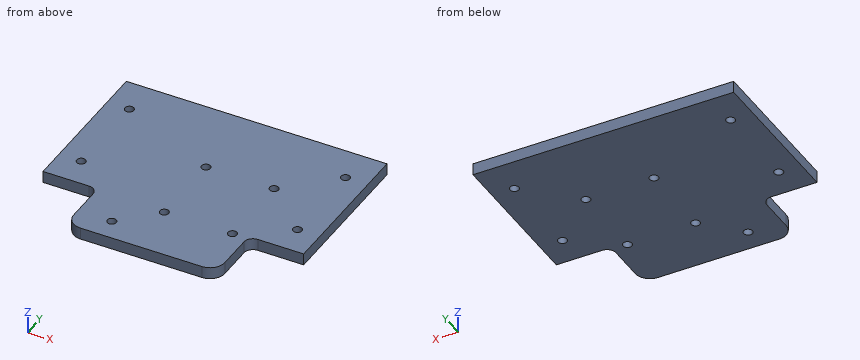
```python
from build123d import *

# Parameters (mm, degrees)
SKETCH_1_W          = 88
SKETCH_1_H          = 72
EXTRUDE_1_DEPTH     = 4
SKETCH_2_W          = 18.5
SKETCH_2_H          = 20
CUT_EXTRUDE_1_DEPTH = 114.771701227
FILLET_1_R          = 3
SKETCH_3_W          = 18.5
SKETCH_3_H          = 20
CUT_EXTRUDE_2_DEPTH = 114.771701227
FILLET_2_R          = 3
SKETCH_5_R          = 1.5
CUT_EXTRUDE_4_DEPTH = 114.771701227
SKETCH_4_R          = 1.5
CUT_EXTRUDE_3_DEPTH = 114.771701227
FILLET_4_R          = 5


with BuildPart() as part:
    # 草图1 → 凸台-拉伸1 (new body)
    with BuildSketch(Plane.XY):
        with Locations((44, 36)):
            Rectangle(SKETCH_1_W, SKETCH_1_H)
    extrude(amount=EXTRUDE_1_DEPTH)

    # 草图2 → 切除-拉伸1 (cut, through all)
    with BuildSketch(Plane.XY.offset(4)):
        with Locations((9.25, 10)):
            Rectangle(SKETCH_2_W, SKETCH_2_H)
    extrude(amount=-CUT_EXTRUDE_1_DEPTH, mode=Mode.SUBTRACT)

    # 圆角1
    fillet_1_edges = [part.edges().sort_by_distance(p)[0] for p in [
        (18.5, 20, 2),
    ]]
    fillet(fillet_1_edges, radius=FILLET_1_R)

    # 草图3 → 切除-拉伸2 (cut, through all)
    with BuildSketch(Plane.XY.offset(4)):
        with Locations((78.75, 10)):
            Rectangle(SKETCH_3_W, SKETCH_3_H)
    extrude(amount=-CUT_EXTRUDE_2_DEPTH, mode=Mode.SUBTRACT)

    # 圆角2
    fillet_2_edges = [part.edges().sort_by_distance(p)[0] for p in [
        (69.5, 20, 2),
    ]]
    fillet(fillet_2_edges, radius=FILLET_2_R)

    # 草图5 → 切除-拉伸4 (cut, through all)
    with BuildSketch(Plane.XY.offset(4)):
        with Locations((80.5, 60)):
            Circle(SKETCH_5_R)
        with Locations((80.5, 30)):
            Circle(SKETCH_5_R)
        with Locations(Location((30, 7.5, 0), (0, 0, 180))):
            Circle(SKETCH_5_R)
        with Locations(Location((7.5, 30, 0), (0, 0, 180))):
            Circle(SKETCH_5_R)
        with Locations(Location((7.5, 60, 0), (0, 0, 180))):
            Circle(SKETCH_5_R)
    extrude(amount=-CUT_EXTRUDE_4_DEPTH, mode=Mode.SUBTRACT)

    # 草图4 → 切除-拉伸3 (cut, through all)
    with BuildSketch(Plane.XY.offset(4)):
        with Locations((41.5, 45)):
            Circle(SKETCH_4_R)
        with Locations((64.5, 45)):
            Circle(SKETCH_4_R)
        with Locations((64.5, 19)):
            Circle(SKETCH_4_R)
        with Locations((41.5, 19)):
            Circle(SKETCH_4_R)
    extrude(amount=-CUT_EXTRUDE_3_DEPTH, mode=Mode.SUBTRACT)

    # 圆角4
    fillet_4_edges = [part.edges().sort_by_distance(p)[0] for p in [
        (18.5, 0, 2),
        (69.5, 0, 2),
    ]]
    fillet(fillet_4_edges, radius=FILLET_4_R)


solid = part.part
```
CAD build for the part. Positions are in the model's coordinates, mm. Round coordinates to 2 decimals unless told otherwise and drop trailing zeros. Order: outer loops, then holes, each group sorted by start corner. A loop starts at its lowest first (then second) coordinate and runs counter-clockwise, first axis right, second up.
Q1. Slice it at D-D (x = 41.5). Write the cut outline in (y, z), and give its area (3 significant figures).
Q2. Slice it at C-C (y = 45). Write the cut outline in (x, z).
Q3. Drop flat-ended pins along their axis: pin 1 (10 mm diameter, centred on x = 19.5, y = 27.5, fed in from -Z); pin 2 (2.5 mm diameter, centred on x = 64.5, y = 19, fed in from -Z); pin 3 (2 mm diameter, centred on x = 4, z = 2, fed in from -Y); pin 4 (2 mm diameter, centred on y = 13, z = 1.5, fed in from +X). Give the stop position or say it passes through.
Q4. Wall check: L1, parallel to Y at x = 64.5, z = 1.95; L2, parallel to Y at x = 7.5, z = 2; L3, parallel to Y at x = 30, z = 3.05. Give the ranges that are in metal, low to high.
Q5. Slice it at B-B (z = 1.55). State how many separate pieces and enclosed holes the cut face has, and give its area (3 significant figures).
Q6. Slice it at A-A (x = 30). Write the cut outline in (y, z), and give its area (3 significant figures).
Results below:
1. outline: (0, 0) - (17.5, 0) - (17.5, 4) - (0, 4) - close; (20.5, 0) - (43.5, 0) - (43.5, 4) - (20.5, 4) - close; (46.5, 0) - (72, 0) - (72, 4) - (46.5, 4) - close
1. area: 264 mm2
2. outline: (0, 0) - (40, 0) - (40, 4) - (0, 4) - close; (43, 0) - (63, 0) - (63, 4) - (43, 4) - close; (66, 0) - (88, 0) - (88, 4) - (66, 4) - close
3. pin 1: stops at z = 0
3. pin 2: passes through
3. pin 3: stops at y = 20
3. pin 4: stops at x = 69.5
4. L1: y = 0 to 17.5, 20.5 to 43.5, 46.5 to 72
4. L2: y = 20 to 28.5, 31.5 to 58.5, 61.5 to 72
4. L3: y = 0 to 6, 9 to 72
5. separate pieces: 1
5. enclosed holes: 9
5. area: 5,530 mm2
6. outline: (0, 0) - (6, 0) - (6, 4) - (0, 4) - close; (9, 0) - (72, 0) - (72, 4) - (9, 4) - close
6. area: 276 mm2
